from build123d import *

# Parameters (mm, degrees)
BOSS_EXTRUDE1_DEPTH             = 2.5
SKETCH3_R                       = 2.25
CUT_EXTRUDE1_DEPTH              = 6
SKETCH4_W                       = 4.5
SKETCH4_H                       = 25
BOSS_EXTRUDE2_DEPTH             = 38
FILLET2_R                       = 2
TAP_DRILL_FOR_M3X0_5_TAP1_D     = 2.5
TAP_DRILL_FOR_M3X0_5_TAP1_DEPTH = 15
TAP_DRILL_FOR_M3X0_5_TAP1_TIP   = 0.751075774
SKETCH4_3_R                     = 1.5
BOSS_EXTRUDE3_DEPTH             = 20
SKETCH8_W                       = 21
SKETCH8_H                       = 7.693946087
SKETCH8_R                       = 3
BOSS_EXTRUDE4_DEPTH             = 25
FILLET3_R                       = 3
FILLET3_OF_MIRROR1_R            = 3
SKETCH9_W                       = 49.73363163
SKETCH9_H                       = 6.646102353
BOSS_EXTRUDE5_DEPTH             = 14
FILLET5_R                       = 3
FILLET6_R                       = 1
SKETCH10_R                      = 1.85
CUT_EXTRUDE2_DEPTH              = 22


with BuildPart() as part:
    # Sketch1 → Boss-Extrude1 (new body, symmetric)
    with BuildSketch(Plane.XY):
        with BuildLine():
            Line((60, 0), (-60, 0))
            Line((-60, 0), (-60, 80))
            ThreePointArc((-60, 80), (0, 100), (60, 80))
            Line((60, 80), (60, 0))
        make_face()
    extrude(amount=BOSS_EXTRUDE1_DEPTH, both=True)

    # Sketch3 → Cut-Extrude1 (cut, through all)
    with BuildSketch(Plane.XY.offset(2.5)):
        with Locations((-52.5, 9)):
            Circle(SKETCH3_R)
        with Locations((-27.5, 9)):
            Circle(SKETCH3_R)
        with Locations((27.5, 9)):
            Circle(SKETCH3_R)
        with Locations((52.5, 9)):
            Circle(SKETCH3_R)
    extrude(amount=-CUT_EXTRUDE1_DEPTH, mode=Mode.SUBTRACT)

    # Sketch4 → Boss-Extrude2 (add)
    with BuildSketch(Plane.XY.offset(2.5)):
        with Locations((46.25, 42.5)):
            Rectangle(SKETCH4_W, SKETCH4_H)
        with Locations((-46.25, 42.5)):
            Rectangle(SKETCH4_W, SKETCH4_H)
    extrude(amount=BOSS_EXTRUDE2_DEPTH)

    # Fillet2
    fillet2_edges = [part.edges().sort_by_distance(p)[0] for p in [
        (46.25, 55, 2.5),
        (44, 42.5, 2.5),
        (48.5, 42.5, 2.5),
        (46.25, 30, 2.5),
        (-48.5, 42.5, 2.5),
        (-46.25, 30, 2.5),
        (-46.25, 55, 2.5),
        (-44, 42.5, 2.5),
    ]]
    fillet(fillet2_edges, radius=FILLET2_R)

    # Tap Drill for M3x0.5 Tap1
    with Locations(Plane.XY.offset(40.5)):
        with Locations((-46.25, 42.5), (46.25, 42.5)):
            Hole(TAP_DRILL_FOR_M3X0_5_TAP1_D / 2, depth=TAP_DRILL_FOR_M3X0_5_TAP1_DEPTH)
            with Locations((0, 0, -(TAP_DRILL_FOR_M3X0_5_TAP1_DEPTH + TAP_DRILL_FOR_M3X0_5_TAP1_TIP / 2))):  # 118° drill point
                Cone(0, TAP_DRILL_FOR_M3X0_5_TAP1_D / 2, TAP_DRILL_FOR_M3X0_5_TAP1_TIP, mode=Mode.SUBTRACT)

    # Sketch4<3> → Boss-Extrude3 (add)
    with BuildSketch(Plane.XY.offset(2.5)):
        with Locations((-15, 22)):
            Circle(SKETCH4_3_R)
        with Locations((15, 22)):
            Circle(SKETCH4_3_R)
        with Locations((-15, 63)):
            Circle(SKETCH4_3_R)
        with Locations((15, 63)):
            Circle(SKETCH4_3_R)
    extrude(amount=BOSS_EXTRUDE3_DEPTH)

    # Sketch8 → Boss-Extrude4 (add)
    with BuildSketch(Plane(origin=(60, 0, 0), x_dir=(0, 0, -1), z_dir=(1, 0, 0))):
        with Locations((8, 74.474861351)):
            Rectangle(SKETCH8_W, SKETCH8_H)
        with Locations((14.5, 74.474861351)):
            Circle(SKETCH8_R, mode=Mode.SUBTRACT)
    boss_extrude4 = extrude(amount=-BOSS_EXTRUDE4_DEPTH)

    # Fillet3
    fillet3_edges = [part.edges().sort_by_distance(p)[0] for p in [
        (47.5, 70.627888307, -2.5),
        (47.5, 78.321834394, -2.5),
        (47.5, 78.321834394, -18.5),
        (47.5, 70.627888307, -18.5),
    ]]
    fillet(fillet3_edges, radius=FILLET3_R)

    # Mirror1: Boss-Extrude4 across plane
    add(boss_extrude4.mirror(Plane(origin=(0, 0, 0), x_dir=(0, 0, 1), z_dir=(1, 0, 0))))

    # Fillet3 of Mirror1
    fillet3_of_mirror1_edges = [part.edges().sort_by_distance(p)[0] for p in [
        (-47.5, 70.627888307, -2.5),
        (-47.5, 78.321834394, -2.5),
        (-47.5, 78.321834394, -18.5),
        (-47.5, 70.627888307, -18.5),
    ]]
    fillet(fillet3_of_mirror1_edges, radius=FILLET3_OF_MIRROR1_R)

    # Sketch9 → Boss-Extrude5 (add)
    with BuildSketch(Plane.XY.offset(2.5)):
        with Locations((0, 82.579227225)):
            Rectangle(SKETCH9_W, SKETCH9_H)
    extrude(amount=BOSS_EXTRUDE5_DEPTH)

    # Fillet5
    fillet5_edges = [part.edges().sort_by_distance(p)[0] for p in [
        (60, 80, -0.153453135),
        (-60, 80, -0.153453135),
    ]]
    fillet(fillet5_edges, radius=FILLET5_R)

    # Fillet6
    fillet6_edges = [part.edges().sort_by_distance(p)[0] for p in [
        (60, 0, 0),
        (-60, 0, 0),
    ]]
    fillet(fillet6_edges, radius=FILLET6_R)

    # Sketch10 → Cut-Extrude2 (cut, through all)
    with BuildSketch(Plane.XY.offset(2.5)):
        with Locations((49, 80)):
            Circle(SKETCH10_R)
        with Locations((49, 65)):
            Circle(SKETCH10_R)
        with Locations((-49, 65)):
            Circle(SKETCH10_R)
        with Locations((-49, 80)):
            Circle(SKETCH10_R)
    extrude(amount=-CUT_EXTRUDE2_DEPTH, mode=Mode.SUBTRACT)


solid = part.part
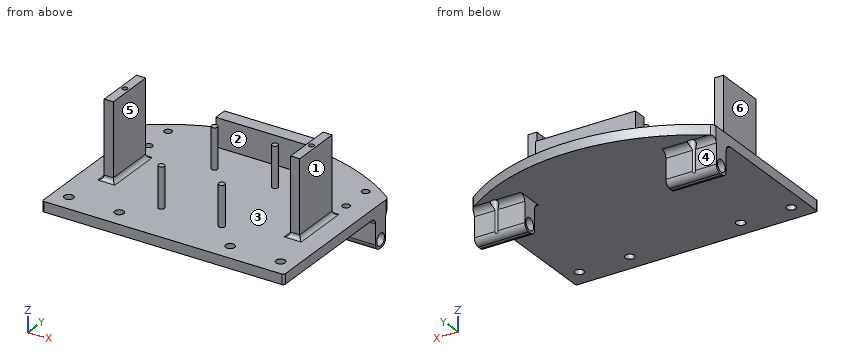
Design review of the part built by this model. Coordinates are the model's own, in mm. Face numbers are marked on the shaded views. A direction names the side the tool comes from. Coordinates: 2 decimals unless noted, no trailing zeros. Order: outer loops, then holes, each group sorted by start corner. A loop starts at its lowest first (then second) coordinate and runs counter-clockwise, first axis right, second up.
Item 1: For pin 1 Ø1.5 at (x, y) = (-15, 63) entering from +Z; pin 2 Ø8 at (x, z) = (-15, 13) entering from +Y; pin 3 Ø7 at (x, z) = (3, 12) entering from -Y, all flat-tipped, find the tip position at first contact; note any pin that passes through.
Item 2: Take a section at B-B, the plane z = -7. Write out the cut boundary in (x, y).
Item 3: Take a section at A-A, the plane z = 28.5. Write out the cut boundary in (x, y), then the cut area to 3 significant figures.
Item 4: The part is to be moulded in two halves that separate along X. For the marked faces 1, 2 and 3, say which applies: pulls with the +X half, pulls with the -X half, needs draft (parallel to the pull), parting line crosses it, or undercut.
Item 5: Take a section at D-D, the plane x = -27.5. Write out the cut boundary in (y, z), then the cut area to 3 significant figures.
Item 6: For line 1 (X direction, y = 42.5, z = 37.75); line 2 (X direction, y = 65, z = 1); line 3 (X direction, y = 42, z = 35), list the stretches that pass through material, from the lowest coordinate up.
Item 7: Take a section at C-C, the plane y = 32.5. Write out the cut boundary in (x, z).
Item 8: For the marked faces 4, 5 and 6, list the 3-axis set-ups (+Z, -Z, +X, -X, +Y, -Y) from which the entire face can be reached by the end or side of a thin tool; tool diameter is ignored.
The answers:
1. pin 1: stops at z = 22.5
1. pin 2: stops at y = 85.9
1. pin 3: stops at y = 79.26
2. outline: (-60, 70.63) - (-35, 70.63) - (-35, 78.32) - (-48.22, 78.32) arc R1.85 cw to (-49.78, 78.32) - (-60, 78.32) - close; (35, 70.63) - (60, 70.63) - (60, 78.32) - (49.78, 78.32) arc R1.85 cw to (48.22, 78.32) - (35, 78.32) - close
3. outline: (-48.5, 30) - (-44, 30) - (-44, 55) - (-48.5, 55) - close; (44, 30) - (48.5, 30) - (48.5, 55) - (44, 55) - close; hole circle Ø2.5 at (-46.25, 42.5); hole circle Ø2.5 at (46.25, 42.5)
3. area: 215 mm2
4. face 1: pulls with the +X half
4. face 2: needs draft
4. face 3: undercut
5. outline: (0, -2.5) - (6.75, -2.5) - (6.75, 2.5) - (0, 2.5) - close; (11.25, -2.5) - (96.14, -2.5) - (96.14, 2.5) - (11.25, 2.5) - close
5. area: 458 mm2
6. line 1: x = -48.5 to -47.5, -45 to -44, 44 to 45, 47.5 to 48.5
6. line 2: x = -60 to -50.85, -47.15 to 47.15, 50.85 to 60
6. line 3: x = -48.5 to -47.4, -45.1 to -44, 44 to 45.1, 47.4 to 48.5
7. outline: (-60, -2.5) - (60, -2.5) - (60, 2.5) - (50.5, 2.5) arc R2 cw to (48.5, 4.5) - (48.5, 40.5) - (44, 40.5) - (44, 4.5) arc R2 cw to (42, 2.5) - (-42, 2.5) arc R2 cw to (-44, 4.5) - (-44, 40.5) - (-48.5, 40.5) - (-48.5, 4.5) arc R2 cw to (-50.5, 2.5) - (-60, 2.5) - close
8. face 4: -Z, +X, -X, +Y
8. face 5: +Z, +Y, -Y
8. face 6: +Z, -X, +Y, -Y
